from build123d import *

# Parameters (mm, degrees)
SKETCH1_W           = 46.1
SKETCH1_H           = 26.1
SKETCH1_W_2         = 40.1
SKETCH1_H_2         = 20.1
BOSS_EXTRUDE1_DEPTH = 28
SKETCH2_W           = 46.1
SKETCH2_H           = 26.1
BOSS_EXTRUDE2_DEPTH = 3
SKETCH3_W           = 3.95
SKETCH3_H           = 26.1
BOSS_EXTRUDE3_DEPTH = 5
SKETCH4_R           = 1
CUT_EXTRUDE1_DEPTH  = 13
SKETCH5_R           = 10
BOSS_EXTRUDE4_DEPTH = 2
SKETCH7_W           = 3
SKETCH7_H           = 26
BOSS_EXTRUDE5_DEPTH = 5
SKETCH8_W           = 55.2
SKETCH8_H           = 26
BOSS_EXTRUDE6_DEPTH = 5
BOSS_EXTRUDE7_DEPTH = 55.2
SKETCH12_R          = 2.5
SKETCH12_R_2        = 1
CUT_EXTRUDE2_DEPTH  = 13.2
SKETCH13_R          = 10.1
CUT_EXTRUDE3_DEPTH  = 13.2
SKETCH14_W          = 47.2
SKETCH14_H          = 32
CUT_EXTRUDE4_DEPTH  = 43.2
SKETCH15_R          = 10.1
CUT_EXTRUDE5_DEPTH  = 2.8
SKETCH16_W          = 4
SKETCH16_H          = 6
CUT_EXTRUDE6_DEPTH  = 24


with BuildPart() as part:
    # Sketch1 → Boss-Extrude1 (new body)
    with BuildSketch(Plane.XY):
        Rectangle(SKETCH1_W, SKETCH1_H)
        Rectangle(SKETCH1_W_2, SKETCH1_H_2, mode=Mode.SUBTRACT)
    extrude(amount=BOSS_EXTRUDE1_DEPTH)

    # Sketch2 → Boss-Extrude2 (add)
    with BuildSketch(Plane(origin=(0, 0, 0), x_dir=(-1, 0, 0), z_dir=(0, 0, -1))):
        Rectangle(SKETCH2_W, SKETCH2_H)
    extrude(amount=BOSS_EXTRUDE2_DEPTH)

    # Sketch3 → Boss-Extrude3 (add)
    with BuildSketch(Plane.XY.offset(28)):
        with Locations((-25.025, 0)):
            Rectangle(SKETCH3_W, SKETCH3_H)
        with Locations((25.025, 0)):
            Rectangle(SKETCH3_W, SKETCH3_H)
    extrude(amount=-BOSS_EXTRUDE3_DEPTH)

    # Sketch4 → Cut-Extrude1 (cut)
    with BuildSketch(Plane.XY.offset(28)):
        with Locations((24.4, 5)):
            Circle(SKETCH4_R)
        with Locations((24.4, -5)):
            Circle(SKETCH4_R)
    cut_extrude1 = extrude(amount=-CUT_EXTRUDE1_DEPTH, mode=Mode.SUBTRACT)

    # Mirror1: Cut-Extrude1 across plane
    add(cut_extrude1.mirror(Plane(origin=(0, 0, 0), x_dir=(0, 0, 1), z_dir=(1, 0, 0))), mode=Mode.SUBTRACT)

    # Sketch5 → Boss-Extrude4 (add)
    with BuildSketch(Plane(origin=(0, 0, -3), x_dir=(-1, 0, 0), z_dir=(0, 0, -1))):
        with Locations((10.05, 0)):
            Circle(SKETCH5_R)
    extrude(amount=BOSS_EXTRUDE4_DEPTH)

    # Sketch7 → Boss-Extrude5 (add)
    with BuildSketch(Plane(origin=(0, 13.05, 0), x_dir=(1, 0, 0), z_dir=(0, 1, 0))):
        with Locations((-20.05, -10)):
            Rectangle(SKETCH7_W, SKETCH7_H)
        with Locations((-10.05, -10)):
            Rectangle(SKETCH7_W, SKETCH7_H)
        with Locations((-0.05, -10)):
            Rectangle(SKETCH7_W, SKETCH7_H)
        with Locations((9.95, -10)):
            Rectangle(SKETCH7_W, SKETCH7_H)
        with Locations((19.95, -10)):
            Rectangle(SKETCH7_W, SKETCH7_H)
    extrude(amount=BOSS_EXTRUDE5_DEPTH)

    # Sketch8 → Boss-Extrude6 (add)
    with BuildSketch(Plane(origin=(0, 18.05, 0), x_dir=(1, 0, 0), z_dir=(0, 1, 0))):
        with Locations((0, -10)):
            Rectangle(SKETCH8_W, SKETCH8_H)
    extrude(amount=BOSS_EXTRUDE6_DEPTH)

    # Sketch9 → Boss-Extrude7 (add)
    with BuildSketch(Plane.ZY.offset(27.6)):
        with BuildLine():
            Line((-3, 23.05), (-1.985460019, 43.640549012))
            ThreePointArc((-1.985460019, 43.640549012), (10, 55.05), (21.985460019, 43.640549012))
            Line((21.985460019, 43.640549012), (23, 23.05))
            Line((23, 23.05), (-3, 23.05))
        make_face()
    extrude(amount=-BOSS_EXTRUDE7_DEPTH)

    # Sketch12 → Cut-Extrude2 (cut)
    with BuildSketch(Plane.ZY.offset(27.6)):
        with Locations((10, 43.05)):
            Circle(SKETCH12_R)
        with Locations((10, 50.05)):
            Circle(SKETCH12_R_2)
        with Locations((13, 50.05)):
            Circle(SKETCH12_R_2)
        with Locations((7, 50.05)):
            Circle(SKETCH12_R_2)
        with Locations((17, 46.05)):
            Circle(SKETCH12_R_2)
        with Locations((17, 43.05)):
            Circle(SKETCH12_R_2)
        with Locations((17, 40.05)):
            Circle(SKETCH12_R_2)
        with Locations((13, 36.05)):
            Circle(SKETCH12_R_2)
        with Locations((10, 36.05)):
            Circle(SKETCH12_R_2)
        with Locations((7, 36.05)):
            Circle(SKETCH12_R_2)
        with Locations((3, 40.05)):
            Circle(SKETCH12_R_2)
        with Locations((3, 43.05)):
            Circle(SKETCH12_R_2)
        with Locations((3, 46.05)):
            Circle(SKETCH12_R_2)
    extrude(amount=-CUT_EXTRUDE2_DEPTH, mode=Mode.SUBTRACT)

    # Sketch13 → Cut-Extrude3 (cut)
    with BuildSketch(Plane(origin=(27.6, 0, 0), x_dir=(0, 0, -1), z_dir=(1, 0, 0))):
        with Locations((-10, 43.05)):
            Circle(SKETCH13_R)
    extrude(amount=-CUT_EXTRUDE3_DEPTH, mode=Mode.SUBTRACT)

    # Sketch14 → Cut-Extrude4 (cut)
    with BuildSketch(Plane(origin=(0, 0, -3), x_dir=(-1, 0, 0), z_dir=(0, 0, -1))):
        with Locations((-1, 39.05)):
            Rectangle(SKETCH14_W, SKETCH14_H)
    extrude(amount=-CUT_EXTRUDE4_DEPTH, mode=Mode.SUBTRACT)

    # Sketch15 → Cut-Extrude5 (cut)
    with BuildSketch(Plane(origin=(-22.6, 0, 0), x_dir=(0, 0, -1), z_dir=(1, 0, 0))):
        with Locations((-10, 43.05)):
            Circle(SKETCH15_R)
    extrude(amount=-CUT_EXTRUDE5_DEPTH, mode=Mode.SUBTRACT)

    # Sketch16 → Cut-Extrude6 (cut)
    with BuildSketch(Plane.XY.offset(28)):
        with Locations((-22.05, 0)):
            Rectangle(SKETCH16_W, SKETCH16_H)
    extrude(amount=-CUT_EXTRUDE6_DEPTH, mode=Mode.SUBTRACT)


solid = part.part
Source: CAD feature listing. Evaluate the final solid. Frame: model axes, mm. A direction names the side the tool comes from. Round coordinates to 2 decimals unless told otherwise and drop trailing zeros. Order: outer loops, then holes, each group sorted by start corner. A loop starts at its lowest first (then second) coordinate and runs counter-clockwise, first axis right, second up. Notation, with made-up numbers: (9.5, 33.25) - (65.5, 33.25) arc R29 ccw to (65.5, 54.25) - close; hole circle Ø7 at (72, 60). An arc over 180 degrees is marked (long way). Use a Markdown table: item, result. Add a question column.
1. Section query B-B (x = 15.5). Return the cut outline in (y, z).
2. Section query D-D (x = -10.05). Return the cut outline in (y, z), then the cut area to 3 significant figures.
3. Set-up query: faces 4 (the flat face through (-21.55, 16, 10)), 5 (the flat face through (-8.55, 16, 10)), 6 (the flat face through (25, 0, 23)), 7 (the flat face through (0, -10.05, 14)), 8 (the cylindrical face through (-26.515, 35.074, 6.783)). Return all of +Z, -Z, +X, -X, +Y, -Y with unobstructed straight access to the full face (end or side cutting, diameter ignored); none if empty.
4. Line query: probe 1 along Y at (x, z) = (-8.5, 19.5); probe 2 along Y at (x, z) = (-24.4, 24.2); probe 3 along Y at (x, z) = (-26.8, 10). Output: solid intervals per line, ascending.
5. Mould query, pull axis Z, two halves, no side actions, for faces 1 (the cylindrical face through (-26.515, 49.074, 12.783)), 2 (the flat face through (0, 0, 0)), 3 (the flat face through (27.6, 32.7, 10.2)). Classes: +Z half, -Z half, draft (parallel to the pull), parting line (faces both ways), or undercut.
6. Section query A-A (y = 0). Return the cut outline in (x, z), then the cut area to 3 significant figures.
7. Section query C-C (y = 15.5). Return the cut outline in (x, z), then the cut area to 3 significant figures.
8. First-contact query: pin 1 (1.8 mm diameter, centred on y = 36.05, z = 7, fed in from -X); pin 2 (3 mm diameter, centred on x = 14.5, z = 2.5, fed in from +Y); pin 3 (3 mm diameter, centred on y = 36.05, z = 10, fed in from +X); pin 4 (5.5 mm diameter, centred on y = 14.5, z = 10, fed in from +X). Flat tips, straight axial feed; report the tip coordinate or a pass-through.
Derived:
| question | item | result |
|---|---|---|
| 1 | outline | (-13.05, -3) - (13.05, -3) - (13.05, 28) - (10.05, 28) - (10.05, 0) - (-10.05, 0) - (-10.05, 28) - (-13.05, 28) - close; (18.05, -3) - (23.05, -3) - (23.05, 23) - (18.05, 23) - close |
| 2 | outline | (-13.05, -3) - (-10, -3) - (-10, -5) - (10, -5) - (10, -3) - (23.05, -3) - (23.05, 23) - (13.05, 23) - (13.05, 28) - (10.05, 28) - (10.05, 0) - (-10.05, 0) - (-10.05, 28) - (-13.05, 28) - close |
| 2 | area | 546 mm2 |
| 3 | face 4 | +Z, -Z, -X |
| 3 | face 5 | +Z, -Z |
| 3 | face 6 | -Z, +X, -Y |
| 3 | face 7 | +Z |
| 3 | face 8 | +X, -X |
| 4 | probe 1 | -13.05 to -10.05, 10.05 to 13.05, 18.05 to 23.05 |
| 4 | probe 2 | -13.05 to -6, -4 to 4, 6 to 13.05 |
| 4 | probe 3 | 18.05 to 35.05, 37.05 to 40.55, 45.55 to 49.05, 51.05 to 55.05 |
| 5 | face 1 | undercut |
| 5 | face 2 | +Z half |
| 5 | face 3 | draft |
| 6 | outline | (-27, 23) - (-24.05, 23) - (-24.05, 28) - (-27, 28) - close; (-23.05, -3) - (-20.05, -3) - (-20.05, -5) - (-0.05, -5) - (-0.05, -3) - (23.05, -3) - (23.05, 23) - (27, 23) - (27, 28) - (20.05, 28) - (20.05, 0) - (-20.05, 0) - (-20.05, 4) - (-23.05, 4) - close |
| 6 | area | 309 mm2 |
| 7 | outline | (-21.55, -3) - (-18.55, -3) - (-18.55, 23) - (-21.55, 23) - close; (-11.55, -3) - (-8.55, -3) - (-8.55, 23) - (-11.55, 23) - close; (-1.55, -3) - (1.45, -3) - (1.45, 23) - (-1.55, 23) - close; (8.45, -3) - (11.45, -3) - (11.45, 23) - (8.45, 23) - close; (18.45, -3) - (21.45, -3) - (21.45, 23) - (18.45, 23) - close |
| 7 | area | 390 mm2 |
| 8 | pin 1 | through |
| 8 | pin 2 | y = 23.05 |
| 8 | pin 3 | x = -25.4 |
| 8 | pin 4 | x = 23.05 |
